Could you check a few things on this model? Use its own coordinates, in mm. Face numbers are marked on the shaded views. A direction names the side the tool comes from. Round coordinates to 2 decimals unless told otherwise and drop trailing zeros. Loops run counter-clockwise (first coordinate to the right, second up) from the corner with the lowest first, then second, coordinate; pieces in that order, holes last. Notation, with made-up numbers: M -3,88 L 9,88 A22 ccw 9,111 Z; hole C 78,41 d10. An arc over 180 degrees is marked long. Answer in a Markdown table with one row per item.
```python
from build123d import *

# Parameters (mm, degrees)
SKETCH1_W           = 80
SKETCH1_H           = 80
SKETCH1_R           = 3
BOSS_EXTRUDE1_DEPTH = 123
SKETCH2_R           = 35
BOSS_EXTRUDE2_DEPTH = 3
SKETCH4_W           = 17
SKETCH4_H           = 17
CUT_EXTRUDE1_DEPTH  = 115
FILLET1_R           = 3


with BuildPart() as part:
    # Sketch1 → Boss-Extrude1 (new body)
    with BuildSketch(Plane.XY):
        Rectangle(SKETCH1_W, SKETCH1_H)
        with Locations((-31.819805153, 31.819805153)):
            Circle(SKETCH1_R, mode=Mode.SUBTRACT)
        with Locations((31.819805153, 31.819805153)):
            Circle(SKETCH1_R, mode=Mode.SUBTRACT)
        with Locations((31.819805153, -31.819805153)):
            Circle(SKETCH1_R, mode=Mode.SUBTRACT)
        with Locations((-31.819805153, -31.819805153)):
            Circle(SKETCH1_R, mode=Mode.SUBTRACT)
    extrude(amount=BOSS_EXTRUDE1_DEPTH)

    # Sketch2 → Boss-Extrude2 (add)
    with BuildSketch(Plane.XY.offset(123)):
        Circle(SKETCH2_R)
    extrude(amount=BOSS_EXTRUDE2_DEPTH)

    # Sketch4 → Cut-Extrude1 (cut)
    with BuildSketch(Plane(origin=(0, 0, 0), x_dir=(-1, 0, 0), z_dir=(0, 0, -1))):
        with Locations((31.5, 31.5)):
            Rectangle(SKETCH4_W, SKETCH4_H)
        with Locations((-31.5, 31.5)):
            Rectangle(SKETCH4_W, SKETCH4_H)
        with Locations((31.5, -31.5)):
            Rectangle(SKETCH4_W, SKETCH4_H)
        with Locations((-31.5, -31.5)):
            Rectangle(SKETCH4_W, SKETCH4_H)
    extrude(amount=-CUT_EXTRUDE1_DEPTH, mode=Mode.SUBTRACT)

    # Fillet1
    fillet1_edges = [part.edges().sort_by_distance(p)[0] for p in [
        (40, -23, 57.5),
        (23, -23, 57.5),
        (23, -40, 57.5),
        (-23, -40, 57.5),
        (-23, -23, 57.5),
        (-40, -23, 57.5),
        (-40, 23, 57.5),
        (-23, 23, 57.5),
        (-23, 40, 57.5),
        (40, 23, 57.5),
        (23, 40, 57.5),
        (23, 23, 57.5),
        (40, -40, 119),
        (-40, -40, 119),
        (-40, 40, 119),
        (40, 40, 119),
    ]]
    fillet(fillet1_edges, radius=FILLET1_R)


solid = part.part
```
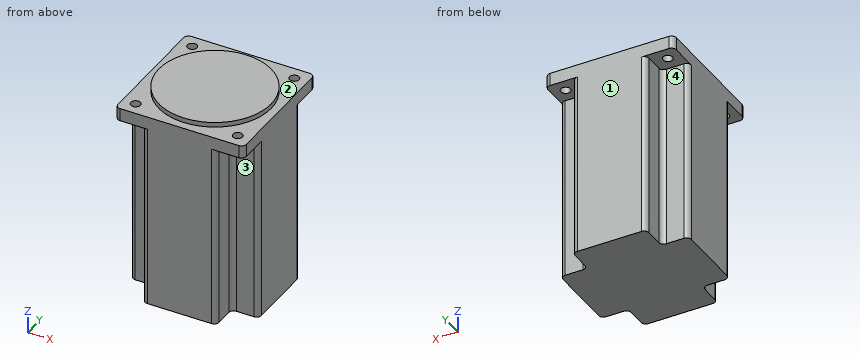
1) I need wall thicknesses on line 1 (Y direction, x = -32, z = 121.5); line 2 (Z direction, x = 34, y = 21.5); line 3 (Z direction, x = -25.5, y = 36). Which ranges of each line are inside material? Lowest first, please.
Computed:
| item | result |
|---|---|
| line 1 | y = -40 to -34.81, -28.83 to 28.83, 34.81 to 40 |
| line 2 | z = 0 to 123 |
| line 3 | z = 115 to 123 |
2) Which directions (+Z, -Z, +X, -X, +Y, -Y) give clear straight access to the entire face, cutting with the end or side of a thin tool? Please do the marked faces 1, 2, 3 and 4.
Computed:
| item | result |
|---|---|
| face 1 | +Z, -Z, +X, -X, +Y |
| face 2 | +Z |
| face 3 | -Z, +X, -Y |
| face 4 | -Z, -X, +Y |
3) Will these pins go through, and if not, where does the flat tip stop? P1, Ø3, axis at x = -26, z = 21.5, coming from the -Y side; P2, Ø2, axis at y = -30.5, z = 78, coming from the +X side; P3, Ø5.5, axis at x = -32, z = 41, coming from the +Y side; P4, Ø5.5, axis at x = -31.82, y = 31.82, coming from the +Z side.
Computed:
| item | result |
|---|---|
| P1 | stops at y = -23.4 |
| P2 | stops at x = 23 |
| P3 | stops at y = 23 |
| P4 | passes through |
4) I want a section at A-A, the plane z = 20. Please give me the cut outline in (x, y), plus the area to 3 significant figures.
Computed:
| item | result |
|---|---|
| outline | M -40,-20 A3 ccw -37,-23 L -26,-23 A3 cw -23,-26 L -23,-37 A3 ccw -20,-40 L 20,-40 A3 ccw 23,-37 L 23,-26 A3 cw 26,-23 L 37,-23 A3 ccw 40,-20 L 40,20 A3 ccw 37,23 L 26,23 A3 cw 23,26 L 23,37 A3 ccw 20,40 L -20,40 A3 ccw -23,37 L -23,26 A3 cw -26,23 L -37,23 A3 ccw -40,20 Z |
| area | 5,240 mm² |
